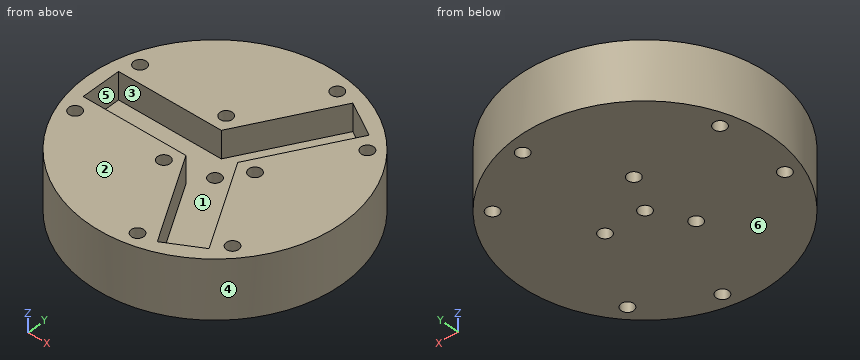
from build123d import *

# Parameters (mm, degrees)
F0_R            = 32.5
F1_DEPTH        = 15
F2_W            = 29
F2_H            = 10
F3_DEPTH        = 7
F3_COPIES_COUNT = 3
F4_R            = 1.5875
F5_DEPTH        = 25.4
F6_R            = 1.5875
F7_DEPTH        = 25.4


# Not quite as in the source:
# - a pattern or mirror of a feature is missing from the dataset's text; its kind, count and spacing are read off the source's solid


with BuildPart() as f1:
    # F0 (on Top) → F1 (new body)
    with BuildSketch(Plane.XY):
        Circle(F0_R)
    extrude(amount=F1_DEPTH)

    # F2 (on face) → F3 (cut)
    with BuildSketch(Plane.XY.offset(15)):
        with Locations((-14.5, 0)):
            Rectangle(F2_W, F2_H)
    f3 = extrude(amount=-F3_DEPTH, mode=Mode.SUBTRACT)

    # F3_copies: F3 ×3 about axis
    f3_copies_axis = Axis((0, 0, 0), (0, 0, 1))
    for i in range(1, F3_COPIES_COUNT):
        add(f3.rotate(f3_copies_axis, i * 360 / F3_COPIES_COUNT), mode=Mode.SUBTRACT)

    # F4 (on face) → F5 (cut)
    with BuildSketch(Plane.XY.offset(8)):
        Circle(F4_R)
    extrude(amount=-F5_DEPTH, mode=Mode.SUBTRACT)

    # F6 (on face) → F7 (cut)
    with BuildSketch(Plane.XY.offset(15)):
        with Locations((10.16, 0)):
            Circle(F6_R)
        with Locations((21.59, 19.05)):
            Circle(F6_R)
        with Locations((21.59, -19.05)):
            Circle(F6_R)
        with Locations((-5.08, 8.7988181024)):
            Circle(F6_R)
        with Locations((5.7027839421, 28.2224884677)):
            Circle(F6_R)
        with Locations((-27.2927839421, 9.1724884677)):
            Circle(F6_R)
        with Locations((-27.2927839421, -9.1724884677)):
            Circle(F6_R)
        with Locations((-5.08, -8.7988181024)):
            Circle(F6_R)
        with Locations((5.7027839421, -28.2224884677)):
            Circle(F6_R)
    extrude(amount=-F7_DEPTH, mode=Mode.SUBTRACT)


solid = f1.part
Read the model definition and answer for the solid it produces. Units are mm, in the model's axes. Face numbers are marked on the shaded views. A direction names the side the tool comes from. Give positions to 0.01 mm unless a question says otherwise; leave off trailing zeros. Write each loop counter-clockwise with the first axis right and the second up, starting at its lowest first coordinate (ties: lowest second). Pieces come first, ordered by that corner, then holes. Notation, with made-up numbers: (-15, -23) - (38, -23) arc R10 cw to (38, -18) - close; hole circle Ø6 at (52.5, 15). An arc over 180 degrees is marked (long way). Use CSV: the item, a comma, the result in double quotes. Start each with the question number.
Item 1: The part is cut by section D-D, the plane y = -19.05. Give the vertices of the cut face in (x, z), and give its area (3 significant figures).
Item 2: For the marked faces 1 and 2, determine the directions among +Z, -Z, +X, -X, +Y, -Y from which every point of the face is accessible in a straight line to the end or side of a thin tool.
Item 3: The mould has two halves that part along X. Classify the marked faces 3, 4, 5 and 6: pulls with the +X half, pulls with the -X half, needs draft (parallel to the pull), parting line crosses it, or undercut.
Item 4: The part is cut by section C-C, the plane x = -27. Give the vertices of the cut face in (y, z).
Item 5: Consider line 1 (Y direction, x = 21.59, z = 6); line 2 (X direction, y = 18.5, z = 8.5); line 3 (Y direction, x = 5, z = 7.5). Determine where each line is inside the solid, lowest interval first.
Item 6: The part is cut by section A-A, the plane x = 0. Give the vertices of the cut face in (y, z).
Item 7: Flat-ended cylindrical pins translate along their axes: P1, Ø5.5, axis at x = -9.5, z = 10.5, coming from the -Y side; P2, Ø3, axis at x = 1, z = 10.5, coming from the +Y side; P3, Ø3, axis at x = 2.5, z = 10.5, coming from the -Y side. Find the tip coordinate at first contact, or state that the pin passes through.
Item 8: The part is cut by section B-B, the plane z = 9. Count the separate pieces of the cut face and the enclosed holes in it, and give its area (3 significant figures).
Taken from the geometry:
1,outline,"(-26.33, 0) - (20, 0) - (20, 15) - (16.77, 15) - (16.77, 8) - (5.23, 8) - (5.23, 15) - (-26.33, 15) - close; (23.18, 0) - (26.33, 0) - (26.33, 15) - (23.18, 15) - close"
1,area,"661 mm2"
2,face 1,"+Z"
2,face 2,"+Z, +X, -X, +Y, -Y"
3,face 3,"undercut"
3,face 4,"parting line crosses it"
3,face 5,"undercut"
3,face 6,"needs draft"
4,outline,"(-18.09, 0) - (-10.73, 0) - (-10.73, 15) - (-18.09, 15) - close; (-7.61, 0) - (7.61, 0) - (7.61, 15) - (5, 15) - (5, 8) - (-5, 8) - (-5, 15) - (-7.61, 15) - close; (10.73, 0) - (18.09, 0) - (18.09, 15) - (10.73, 15) - close"
5,line 1,"-24.29 to -20.64, -17.46 to 17.46, 20.64 to 24.29"
5,line 2,"-26.72 to 4.91, 16.45 to 20.1, 23.08 to 26.72"
5,line 3,"-32.11 to -29.65, -26.8 to 26.8, 29.65 to 32.11"
6,outline,"(-32.5, 0) - (-1.59, 0) - (-1.59, 8) - (-10, 8) - (-10, 15) - (-32.5, 15) - close; (1.59, 0) - (32.5, 0) - (32.5, 15) - (10, 15) - (10, 8) - (1.59, 8) - close"
7,P1,"y = -31.79"
7,P2,"y = 32.5"
7,P3,"y = -32.48"
8,separate pieces,"1"
8,enclosed holes,"10"
8,area,"2,420 mm2"
